Check sheet for the modelled part. Datum: model origin and axes. Units: mm. A direction names the side the tool comes from. Coordinates: 2 decimals unless noted, no trailing zeros. Order: outer loops, then holes, each group sorted by start corner. A loop starts at its lowest first (then second) coordinate and runs counter-clockwise, first axis right, second up.
1. Cross-section at B-B (z = 2). Enter the section's corners in (x, y), then the cut area to 3 significant figures.
2. Cross-section at C-C (y = -2.4). Enter the section's corners in (x, z).
3. Set-up check for faces 5 (the cylindrical face through (0, -4.5, 5.3)), 6 (the flat face through (0, -2, -6.5)): record each of +Z, -Z, +X, -X, +Y, -Y from which the full face is reachable in a straight line by a thin tool's end or side.
4. Cross-section at D-D (z = -1.75). Enter the section's corners in (x, y).
5. Thickness scan on line 1 (Z direction, x = 0, y = -2.55); line 2 (X direction, y = -1.7, z = 3.5); line 3 (X direction, y = -1.8, z = 1). Record the ranges inside material, lowest first.
6. Cross-section at A-A (x = 0). Enter the section's corners in (y, z).
7. Draft check along X on faces 1 (the flat face through (2.7, -2.7, 0.1)), 2 (the cylindrical face through (0, -4.5, -2.1)), 3 (the flat face through (-2.7, -2.7, 0.1)), 4 (the cylindrical face through (-0.969, -2.084, 3.863)). Enter one of: released by +X, released by -X, zero draft, split by the parting line, or undercut.
8. Gauge pin test, flat ends, axial feed: pin 1 Ø3 at (y, z) = (-0.5, -0.5) entering from -X; pin 2 Ø0.6 at (x, z) = (-3.5, -2.5) entering from +Y. Record the tip position at first contact, or that the pin passes through.
```python
from build123d import *

# Parameters (mm, degrees)
EXTRUDE_1_DEPTH             = 6.5
HOLE_WIZARD_M51_D           = 4.2
HOLE_WIZARD_M51_CSINK_D     = 5.2
HOLE_WIZARD_M51_CSINK_ANGLE = 90
FILLET_1_R                  = 0.3


with BuildPart() as part:
    # Эскиз1 → Бобышка-Вытянуть1 (new body, symmetric)
    with BuildSketch(Plane.XY):
        with BuildLine():
            Line((-3, 0), (3, 0))
            Line((3, 0), (3, -0.8))
            Line((3, -0.8), (4, -0.8))
            Line((4, -0.8), (4, -1.4))
            Line((4, -1.4), (1.536396103, -3.863603897))
            ThreePointArc((1.536396103, -3.863603897), (0, -4.5), (-1.536396103, -3.863603897))
            Line((-1.536396103, -3.863603897), (-4, -1.4))
            Line((-4, -1.4), (-4, -0.8))
            Line((-4, -0.8), (-3, -0.8))
            Line((-3, -0.8), (-3, 0))
        make_face()
    extrude(amount=EXTRUDE_1_DEPTH, both=True)

    # Отверстие обработанное метчиком M51 (through all)
    with Locations(Plane(origin=(0, 0, 0), x_dir=(1, 0, 0), z_dir=(0, 1, 0))):
        with Locations((0, -2)):
            CounterSinkHole(HOLE_WIZARD_M51_D / 2, HOLE_WIZARD_M51_CSINK_D / 2, counter_sink_angle=HOLE_WIZARD_M51_CSINK_ANGLE)

    # Эскиз5 → Повернуть1 (revolve)
    with BuildSketch(Plane(origin=(0, 0, 0), x_dir=(0, 0, -1), z_dir=(1, 0, 0))):
        with BuildLine():
            Line((4, -2), (4, -5))
            ThreePointArc((4, -5), (2.5, -3.5), (4, -2))
        make_face()
    revolve(axis=Axis((0, -2, -4), (0, -1, 0)))

    # Скругление1
    fillet_1_edges = [part.edges().sort_by_distance(p)[0] for p in [
        (4, -0.8, 0),
        (4, -1.4, 0),
        (-4, -1.4, 0),
        (-4, -0.8, 0),
    ]]
    fillet(fillet_1_edges, radius=FILLET_1_R)


solid = part.part
```
Data:
1. outline: (-4, -1.28) arc R0.3 ccw to (-3.91, -1.49) - (-2.1, -3.3) - (-2.1, -0.5) - (-2.6, 0) - (-3, 0) - (-3, -0.8) - (-3.7, -0.8) arc R0.3 ccw to (-4, -1.1) - close; (2.1, -3.3) - (3.91, -1.49) arc R0.3 ccw to (4, -1.28) - (4, -1.1) arc R0.3 ccw to (3.7, -0.8) - (3, -0.8) - (3, 0) - (2.6, 0) - (2.1, -0.5) - close
1. area: 7.04 mm2
2. outline: (-3, -6.5) - (3, -6.5) - (3, 6.5) - (-3, 6.5) - close; hole circle Ø4.2 at (0, 2)
3. face 5: +Z, -Y
3. face 6: -Z, +X, -X, +Y, -Y
4. outline: (-4, -1.28) arc R0.3 ccw to (-3.91, -1.49) - (-1.54, -3.86) arc R2.17 ccw to (1.54, -3.86) - (3.91, -1.49) arc R0.3 ccw to (4, -1.28) - (4, -1.1) arc R0.3 ccw to (3.7, -0.8) - (3, -0.8) - (3, 0) - (-3, 0) - (-3, -0.8) - (-3.7, -0.8) arc R0.3 ccw to (-4, -1.1) - close
5. line 1: z = -6.5 to -0.1, 4.1 to 6.5
5. line 2: x = -3.7 to -1.47, 1.47 to 3.7
5. line 3: x = -3.6 to -1.85, 1.85 to 3.6
6. outline: (-4.5, -6.5) - (0, -6.5) - (0, -0.6) - (-0.5, -0.1) - (-4.5, -0.1) - (-4.5, -2.88) arc R1.5 ccw to (-4.5, -5.12) - close; (-4.5, 4.1) - (-0.5, 4.1) - (0, 4.6) - (0, 6.5) - (-4.5, 6.5) - close
7. face 1: released by +X
7. face 2: split by the parting line
7. face 3: released by -X
7. face 4: undercut
8. pin 1: stops at x = -4
8. pin 2: stops at y = -0.8
